```python
from build123d import *

# Parameters (mm, degrees)
SKETCH_1_W          = 86.4
SKETCH_1_H          = 42
EXTRUDE_1_DEPTH     = 2
SKETCH_2_W          = 4.1
SKETCH_2_H          = 40.1
CUT_EXTRUDE_1_DEPTH = 2
SKETCH_4_R          = 1
CUT_EXTRUDE_2_DEPTH = 2
SKETCH_5_R          = 1.55
CUT_EXTRUDE_3_DEPTH = 2
SKETCH_6_R          = 1.55
CUT_EXTRUDE_4_DEPTH = 2
SKETCH_7_W          = 2
SKETCH_7_H          = 30
CUT_EXTRUDE_5_DEPTH = 2
FILLET_1_R          = 1
FILLET_2_R          = 3


with BuildPart() as part:
    # 草图1 → 凸台-拉伸1 (new body)
    with BuildSketch(Plane(origin=(0, 0, 0), x_dir=(1, 0, 0), z_dir=(0, 1, 0))):
        Polygon((-67.2, 28.25), (-74.2, 28.25), (-74.2, -28), (-67.2, -28), (67.8, -28), (67.8, 28.25), align=None)
        Rectangle(SKETCH_1_W, SKETCH_1_H, mode=Mode.SUBTRACT)
    extrude(amount=EXTRUDE_1_DEPTH)

    # 草图2 → 切除-拉伸1 (cut)
    with BuildSketch(Plane(origin=(0, 2, 0), x_dir=(1, 0, 0), z_dir=(0, 1, 0))):
        with Locations((-50.75, 0)):
            Rectangle(SKETCH_2_W, SKETCH_2_H)
        with Locations((50.85, 0)):
            Rectangle(SKETCH_2_W, SKETCH_2_H)
    extrude(amount=-CUT_EXTRUDE_1_DEPTH, mode=Mode.SUBTRACT)

    # 草图4 → 切除-拉伸2 (cut)
    with BuildSketch(Plane(origin=(0, 2, 0), x_dir=(1, 0, 0), z_dir=(0, 1, 0))):
        with Locations((-52.8, 19.05)):
            Circle(SKETCH_4_R)
        with Locations((-48.7, 19.05)):
            Circle(SKETCH_4_R)
        with Locations((-52.8, -19.05)):
            Circle(SKETCH_4_R)
        with Locations((-48.7, -19.05)):
            Circle(SKETCH_4_R)
        with Locations((48.8, -19.05)):
            Circle(SKETCH_4_R)
        with Locations((52.9, -19.05)):
            Circle(SKETCH_4_R)
        with Locations((52.9, 19.05)):
            Circle(SKETCH_4_R)
        with Locations((48.8, 19.05)):
            Circle(SKETCH_4_R)
    extrude(amount=-CUT_EXTRUDE_2_DEPTH, mode=Mode.SUBTRACT)

    # 草图5 → 切除-拉伸3 (cut)
    with BuildSketch(Plane(origin=(0, 2, 0), x_dir=(1, 0, 0), z_dir=(0, 1, 0))):
        with Locations(Location((55.9, 15.05, 0), (0, 0, 270))):
            Circle(SKETCH_5_R)
        with Locations(Location((55.9, 5.05, 0), (0, 0, 270))):
            Circle(SKETCH_5_R)
        with Locations(Location((55.9, -4.95, 0), (0, 0, 270))):
            Circle(SKETCH_5_R)
        with Locations(Location((55.9, -14.95, 0), (0, 0, 270))):
            Circle(SKETCH_5_R)
        with Locations(Location((-55.8, 15.05, 0), (0, 0, 270))):
            Circle(SKETCH_5_R)
        with Locations(Location((-55.8, 5.05, 0), (0, 0, 270))):
            Circle(SKETCH_5_R)
        with Locations(Location((-55.8, -4.95, 0), (0, 0, 270))):
            Circle(SKETCH_5_R)
        with Locations(Location((-55.8, -14.95, 0), (0, 0, 270))):
            Circle(SKETCH_5_R)
    extrude(amount=-CUT_EXTRUDE_3_DEPTH, mode=Mode.SUBTRACT)

    # 草图6 → 切除-拉伸4 (cut)
    with BuildSketch(Plane(origin=(0, 2, 0), x_dir=(1, 0, 0), z_dir=(0, 1, 0))):
        with Locations(Location((57.8, -23, 0), (0, 0, 270))):
            Circle(SKETCH_6_R)
        with Locations(Location((57.8, 23, 0), (0, 0, 90))):
            Circle(SKETCH_6_R)
        with Locations(Location((-67.8, -23, 0), (0, 0, 90))):
            Circle(SKETCH_6_R)
        with Locations(Location((-67.8, 23, 0), (0, 0, 270))):
            Circle(SKETCH_6_R)
    extrude(amount=-CUT_EXTRUDE_4_DEPTH, mode=Mode.SUBTRACT)

    # 草图7 → 切除-拉伸5 (cut)
    with BuildSketch(Plane(origin=(0, 2, 0), x_dir=(1, 0, 0), z_dir=(0, 1, 0))):
        with Locations((-63.2, 0)):
            Rectangle(SKETCH_7_W, SKETCH_7_H)
        with Locations((63.2, 0)):
            Rectangle(SKETCH_7_W, SKETCH_7_H)
    extrude(amount=-CUT_EXTRUDE_5_DEPTH, mode=Mode.SUBTRACT)

    # 圆角1
    fillet_1_edges = [part.edges().sort_by_distance(p)[0] for p in [
        (43.2, 1, 21),
        (43.2, 1, -21),
        (-43.2, 1, -21),
        (-43.2, 1, 21),
    ]]
    fillet(fillet_1_edges, radius=FILLET_1_R)

    # 圆角2
    fillet_2_edges = [part.edges().sort_by_distance(p)[0] for p in [
        (67.8, 1, 28),
        (-74.2, 1, 28),
        (-74.2, 1, -28.25),
        (67.8, 1, -28.25),
    ]]
    fillet(fillet_2_edges, radius=FILLET_2_R)


solid = part.part
```
Source: CAD feature listing. Evaluate the final solid. Frame: model axes, mm. Round coordinates to 2 decimals unless told otherwise and drop trailing zeros. Loops run counter-clockwise (first coordinate to the right, second up) from the corner with the lowest first, then second, coordinate; pieces in that order, holes last.
1. Section query C-C on x = -55.8. Output: boundary loops of the cut face in (y, z), and give its area (3 significant figures).
2. Ray query, L1, parallel to X at y = 1.45, z = 13; L2, parallel to X at y = 1.95, z = 17.5; L3, parallel to Z at x = -67.8, y = 1.05. Return the intervals inside material, ascending.
3. Section query D-D on y = 1.4. Give the number of separate pieces and of enclosed holes in the cut face, and give its area (3 significant figures).
4. Section query B-B on z = -23. Output: boundary loops of the cut face in (x, y).
5. Mould query, pull axis Z, two halves, no side actions, for faces 1 (the cylindrical face through (-54.263, 1.014, -5.252)), 2 (the flat face through (-4, 0, 24)), 3 (the cylindrical face through (-73.34, 1.01, 27.1)). Classes: released by +Z, released by -Z, zero draft, split by the parting line, or undercut.
6. Section query A-A on x = 2. Output: boundary loops of the cut face in (y, z), and give its area (3 significant figures).
Answers below:
1. outline: (0, -28.25) - (2, -28.25) - (2, -16.6) - (0, -16.6) - close; (0, -13.5) - (2, -13.5) - (2, -6.6) - (0, -6.6) - close; (0, -3.5) - (2, -3.5) - (2, 3.4) - (0, 3.4) - close; (0, 6.5) - (2, 6.5) - (2, 13.4) - (0, 13.4) - close; (0, 16.5) - (2, 16.5) - (2, 28) - (0, 28) - close
1. area: 87.7 mm2
2. L1: x = -74.2 to -64.2, -62.2 to -52.8, -48.7 to -43.2, 43.2 to 48.8, 52.9 to 62.2, 64.2 to 67.8
2. L2: x = -74.2 to -52.8, -48.7 to -43.2, 43.2 to 48.8, 52.9 to 67.8
2. L3: z = -28.25 to -24.55, -21.45 to 21.45, 24.55 to 28
3. separate pieces: 1
3. enclosed holes: 17
3. area: 3,800 mm2
4. outline: (-74.2, 0) - (-69.35, 0) - (-69.35, 2) - (-74.2, 2) - close; (-66.25, 0) - (56.25, 0) - (56.25, 2) - (-66.25, 2) - close; (59.35, 0) - (67.8, 0) - (67.8, 2) - (59.35, 2) - close
5. face 1: undercut
5. face 2: zero draft
5. face 3: released by +Z
6. outline: (0, -28.25) - (2, -28.25) - (2, -21) - (0, -21) - close; (0, 21) - (2, 21) - (2, 28) - (0, 28) - close
6. area: 28.5 mm2
